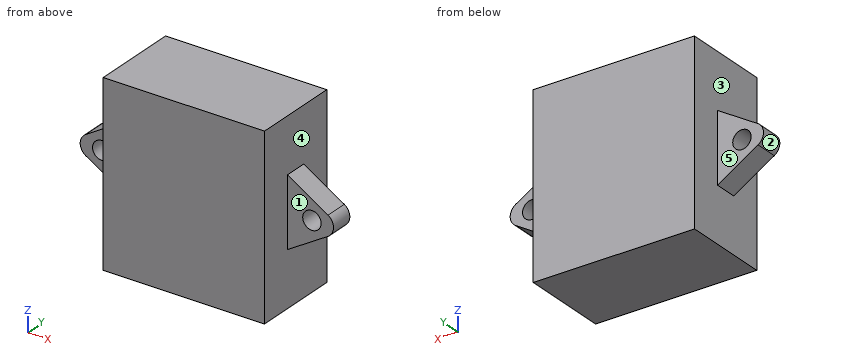
```python
from build123d import *

# Parameters (mm, degrees)
SKETCH_1_W      = 28
SKETCH_1_H      = 31
EXTRUDE_1_DEPTH = 15.3
SKETCH_2_R      = 1.6
EXTRUDE_2_DEPTH = 2


with BuildPart() as part:
    # 草图1 → 凸台-拉伸1 (new body)
    with BuildSketch(Plane(origin=(0, 0, 0), x_dir=(1, 0, 0), z_dir=(0, 1, 0))):
        with Locations((0, -3.201657459)):
            Rectangle(SKETCH_1_W, SKETCH_1_H)
    extrude(amount=EXTRUDE_1_DEPTH)

    # 草图2 → 凸台-拉伸2 (add, symmetric)
    with BuildSketch(Plane(origin=(0, 7.65, 0), x_dir=(1, 0, 0), z_dir=(0, 1, 0))):
        with BuildLine():
            Line((14, 2.798342541), (21.041035209, -1.493955583))
            ThreePointArc((21.041035209, -1.493955583), (22, -3.201657459), (21.041035209, -4.909359334))
            Line((21.041035209, -4.909359334), (14, -9.201657459))
            Line((14, -9.201657459), (14, 2.798342541))
        make_face()
        with Locations(Location((18.25, -3.201657459, 0), (0, 0, 270))):
            Circle(SKETCH_2_R, mode=Mode.SUBTRACT)
    extrude_2 = extrude(amount=EXTRUDE_2_DEPTH, both=True)

    # 镜向1: 凸台-拉伸2 across plane
    add(extrude_2.mirror(Plane(origin=(0, 0, 0), x_dir=(0, 0, 1), z_dir=(1, 0, 0))))


solid = part.part
```
The listing builds one solid part. Answer for the finished solid, in the listing's coordinates (mm). Face numbers are marked on the shaded views. A direction names the side the tool comes from. Coordinates: 2 decimals unless noted, no trailing zeros. Write each loop counter-clockwise with the first axis right and the second up, starting at its lowest first coordinate (ties: lowest second). Pieces come first, ordered by that corner, then holes. Notation, with made-up numbers: (15, 11.25) - (61, 11.25) arc R13 ccw to (61, 19.25) - close; hole circle Ø11 at (76, 24.5). An arc over 180 degrees is marked (long way). Return JSON: item names as keys, results as strings. Group by question number.
Q1. Find the intervals of material crossed by line 1 along X through (y, z) = (10.5, 7.5); line 2 along Y through (x, z) = (15, -2); line 3 along Z through (x, y) = (-18.25, 8.5), in increasing order. Write a range as [from, to].
Q2. Which of the six approach directions +Z, -Z, +X, -X, +Y, -Y give full straight-line access (tool end or side, diameter ignored) to the marked faces 1, 2, 3, 4 and 5?
Q3. Flat-ended cylindrical pins translate along their axes: pin 1 Ø9 at (x, z) = (19, 2) entering from -Y; pin 2 Ø2 at (y, z) = (3, -9) entering from +X; pin 3 Ø6.5 at (x, z) = (-17.5, 3) entering from +Y. Find the tip coordinate at first contact, or state that the pin passes through.
Q4. The part is cut by section A-A on y = 8.5. Write down the section's boundary in (x, z).
Q5. The part is cut by section C-C on z = 15. Write down the section's boundary in (x, y), and give its area (3 significant figures).
Q6. The part is cut by section B-B on x = 17.5. Write down the section's boundary in (y, z).
Q7. The part is cut by section D-D on y = 4.75. Write down the section's boundary in (x, z).
Evaluation:
{
 "1": {"line 1": "x = [-14, 14]", "line 2": "y = [5.65, 9.65]", "line 3": "z = [-0.21, 1.6], [4.8, 6.61]"},
 "2": {"face 1": "+Z, -Z, +X, -Y", "face 2": "-X, +Y, -Y", "face 3": "-X", "face 4": "+X", "face 5": "+Z, -Z, -X, +Y"},
 "3": {"pin 1": "stops at y = 5.65", "pin 2": "stops at x = 14", "pin 3": "stops at y = 9.65"},
 "4": {"outline": "(-21.04, 1.49) - (-14, -2.8) - (-14, -12.3) - (14, -12.3) - (14, -2.8) - (21.04, 1.49) arc R2 ccw to (21.04, 4.91) - (14, 9.2) - (14, 18.7) - (-14, 18.7) - (-14, 9.2) - (-21.04, 4.91) arc R2 ccw to start; hole circle Ø3.2 at (-18.25, 3.2); hole circle Ø3.2 at (18.25, 3.2)"},
 "5": {"outline": "(-14, 0) - (14, 0) - (14, 15.3) - (-14, 15.3) - close", "area": "428 mm2"},
 "6": {"outline": "(5.65, -0.66) - (9.65, -0.66) - (9.65, 1.79) - (5.65, 1.79) - close; (5.65, 4.61) - (9.65, 4.61) - (9.65, 7.07) - (5.65, 7.07) - close"},
 "7": {"outline": "(-14, -12.3) - (14, -12.3) - (14, 18.7) - (-14, 18.7) - close"}
}
